```python
from build123d import *

# Parameters (mm, degrees)
SKETCH1_W           = 13.335
SKETCH1_H           = 2.54
BOSS_EXTRUDE1_DEPTH = 35.56
BOSS_EXTRUDE2_DEPTH = 2.54
CUT_EXTRUDE1_REACH  = 4.54
SKETCH3_R           = 1.905


with BuildPart() as part:
    # Sketch1 → Boss-Extrude1 (new body)
    with BuildSketch(Plane(origin=(0, 0, 0), x_dir=(1, 0, 0), z_dir=(0, 1, 0))):
        Rectangle(SKETCH1_W, SKETCH1_H)
    extrude(amount=BOSS_EXTRUDE1_DEPTH)

    # Sketch2 → Boss-Extrude2 (add)
    with BuildSketch(Plane.XY.offset(1.27)):
        Polygon((-9.2075, 35.56), (-6.6675, 35.56), (6.6675, 35.56), (9.2075, 35.56), (9.2075, 41.91), (-9.2075, 41.91), align=None)
    extrude(amount=-BOSS_EXTRUDE2_DEPTH)

    # Sketch3 → Cut-Extrude1 (cut, up to next)
    with BuildSketch(Plane.XY.offset(1.27), mode=Mode.PRIVATE) as cut_extrude1_sk1:
        with Locations((0, 5.715)):
            Circle(SKETCH3_R)
    cut_extrude1_tool1 = extrude(cut_extrude1_sk1.sketch, amount=-CUT_EXTRUDE1_REACH, mode=Mode.PRIVATE) & part.part
    add(cut_extrude1_tool1.solids().sort_by_distance((0, 5.715, 1.27))[0], mode=Mode.SUBTRACT)
    # Sketch3 → Cut-Extrude1 (cut, up to next)
    with BuildSketch(Plane.XY.offset(1.27), mode=Mode.PRIVATE) as cut_extrude1_sk2:
        with BuildLine():
            Line((1.905, 26.035), (1.905, 22.225))
            ThreePointArc((1.905, 22.225), (0, 20.32), (-1.905, 22.225))
            Line((-1.905, 22.225), (-1.905, 26.035))
            ThreePointArc((-1.905, 26.035), (0, 27.94), (1.905, 26.035))
        make_face()
    cut_extrude1_tool2 = extrude(cut_extrude1_sk2.sketch, amount=-CUT_EXTRUDE1_REACH, mode=Mode.PRIVATE) & part.part
    add(cut_extrude1_tool2.solids().sort_by_distance((0, 24.13, 1.27))[0], mode=Mode.SUBTRACT)


solid = part.part
```
The model under review builds one solid part; all positions refer to its coordinate system, in mm. A direction names the side the tool comes from. Round coordinates to 2 decimals unless told otherwise and drop trailing zeros. Write each loop counter-clockwise with the first axis right and the second up, starting at its lowest first coordinate (ties: lowest second). Pieces come first, ordered by that corner, then holes. Notation, with made-up numbers: (23.5, 66) - (53.5, 66) arc R16 cw to (53.5, 96) - close; hole circle Ø1 at (-19, 80.5). An arc over 180 degrees is marked (long way). Answer as CSV lines item,"result". Start each with the question number.
(1) We need section B-B on z = -0.65. State the section outline as (x, y) points (1 decimal).
(2) For faces 1 (the flat face through (-8, 35.56, 0)), 2 (the flat face through (0, 41.91, 0)), 3 (the flat face through (1.905, 24, 0)), 4 (the flat face through (8, 35.56, 0)), list the 3-axis set-ups (+Z, -Z, +X, -X, +Y, -Y) from which the entire face can be reached by the end or side of a thin tool; tool diameter is ignored.
(3) We need section A-A on x = 0. State the section outline as (y, z) points, plus the area to 3 significant figures.
(4) Draft analysis for pull direction X (two halves, no side actions). For faces 5 (the flat face through (-2, 21, -1.27)), 6 (the flat face through (6.668, 18, 0)), 7 (the cylindrical face through (-0.04, 27.94, 0.02)), 8 (the flat face through (-6.668, 18, 0)), state which applies: pulls with the +X half, pulls with the -X half, needs draft (parallel to the pull), parting line crosses it, or undercut.
(5) We need section C-C on y = 14. State the section outline as (x, z) points, plus the area to 3 significant figures.
(6) For pin 1 Ø1 at (y, z) = (12, 0.5) entering from +X; pin 2 Ø1.3 at (x, z) = (-8, 0.5) entering from -Y; pin 3 Ø3.5 at (x, y) = (0, 5.715) entering from -Z; pin 4 Ø1.3 at (y, z) = (10.5, -0.5) entering from -X, all flat-tipped, find the tip position at first contact; note any pin that passes through.
(7) We need section D-D on x = 8.25. State the section outline as (y, z) points.
(8) To check wall thickness, follow line 1 (Y direction, x = 0, z = 0.55); line 2 (Y direction, x = -0.5, z = 0.35); line 3 (X direction, y = 5, z = -0.1). State the ranges of each line that lie inside material, in increasing order.
Worked answers:
1,outline,"(-9.2, 35.6) - (-6.7, 35.6) - (-6.7, 0) - (6.7, 0) - (6.7, 35.6) - (9.2, 35.6) - (9.2, 41.9) - (-9.2, 41.9) - close; hole circle Ø3.8 at (0, 5.7); hole (-1.9, 22.2) arc R1.9 ccw to (1.9, 22.2) - (1.9, 26) arc R1.9 ccw to (-1.9, 26) - close"
2,face 1,"+Z, -Z, -X, -Y"
2,face 2,"+Z, -Z, +X, -X, +Y"
2,face 3,"+Z, -Z"
2,face 4,"+Z, -Z, +X, -Y"
3,outline,"(0, -1.27) - (3.81, -1.27) - (3.81, 1.27) - (0, 1.27) - close; (7.62, -1.27) - (20.32, -1.27) - (20.32, 1.27) - (7.62, 1.27) - close; (27.94, -1.27) - (41.91, -1.27) - (41.91, 1.27) - (27.94, 1.27) - close"
3,area,"77.4 mm²"
4,face 5,"needs draft"
4,face 6,"pulls with the +X half"
4,face 7,"undercut"
4,face 8,"pulls with the -X half"
5,outline,"(-6.67, -1.27) - (6.67, -1.27) - (6.67, 1.27) - (-6.67, 1.27) - close"
5,area,"33.9 mm²"
6,pin 1,"x = 6.67"
6,pin 2,"y = 35.56"
6,pin 3,"through"
6,pin 4,"x = -6.67"
7,outline,"(35.56, -1.27) - (41.91, -1.27) - (41.91, 1.27) - (35.56, 1.27) - close"
8,line 1,"0 to 3.81, 7.62 to 20.32, 27.94 to 41.91"
8,line 2,"0 to 3.88, 7.55 to 20.39, 27.87 to 41.91"
8,line 3,"-6.67 to -1.77, 1.77 to 6.67"
